from build123d import *

# Parameters (mm, degrees)
SKETCH1_W           = 51.8
SKETCH1_H           = 10.8
BOSS_EXTRUDE1_DEPTH = 12
BOSS_EXTRUDE2_DEPTH = 4
CUT_EXTRUDE1_DEPTH  = 36.675902231
FILLET1_R           = 1
SKETCH4_R           = 3.25
CUT_EXTRUDE2_DEPTH  = 36.675902231
SKETCH5_R           = 4
CUT_EXTRUDE3_DEPTH  = 1.05
M4_TAPPED_HOLE1_D   = 3.3
SKETCH8_R           = 1.25
CUT_EXTRUDE4_DEPTH  = 33.723233337
M4_TAPPED_HOLE2_D   = 3.3


with BuildPart() as part:
    # Sketch1 → Boss-Extrude1 (new body)
    with BuildSketch(Plane.XY):
        Rectangle(SKETCH1_W, SKETCH1_H)
    extrude(amount=BOSS_EXTRUDE1_DEPTH)

    # Sketch2 → Boss-Extrude2 (add)
    with BuildSketch(Plane.XY.offset(12)):
        with BuildLine():
            Line((-25.9, 14.9), (-25.9, 5.4))
            Line((-25.9, 5.4), (-12.9, 5.4))
            Line((-12.9, 5.4), (-12.9, 14.9))
            ThreePointArc((-12.9, 14.9), (-19.4, 21.4), (-25.9, 14.9))
        make_face()
    extrude(amount=-BOSS_EXTRUDE2_DEPTH)

    # Sketch3 → Cut-Extrude1 (cut, through all)
    with BuildSketch(Plane(origin=(0, 0, 0), x_dir=(-1, 0, 0), z_dir=(0, 0, -1))):
        with BuildLine():
            Line((-22.160417654, 0.869411765), (-25.9, 3.1))
            Line((-25.9, 3.1), (-25.9, -5.4))
            Line((-25.9, -5.4), (-18.6, -5.4))
            ThreePointArc((-18.6, -5.4), (-19.552207032, -1.795069427), (-22.160417654, 0.869411765))
        make_face()
    extrude(amount=-CUT_EXTRUDE1_DEPTH, mode=Mode.SUBTRACT)

    # Fillet1
    fillet1_edges = [part.edges().sort_by_distance(p)[0] for p in [
        (-25.9, 5.4, 4),
        (-12.9, 5.4, 10),
        (18.6, -5.4, 6),
        (25.9, 3.1, 6),
        (-25.9, -5.4, 6),
    ]]
    fillet(fillet1_edges, radius=FILLET1_R)

    # Sketch4 → Cut-Extrude2 (cut, through all)
    with BuildSketch(Plane(origin=(0, 0, 0), x_dir=(-1, 0, 0), z_dir=(0, 0, -1))):
        with Locations((20.65, 0.15)):
            Circle(SKETCH4_R)
    extrude(amount=-CUT_EXTRUDE2_DEPTH, mode=Mode.SUBTRACT)

    # Sketch5 → Cut-Extrude3 (cut)
    with BuildSketch(Plane(origin=(0, 0, 0), x_dir=(-1, 0, 0), z_dir=(0, 0, -1))):
        with Locations((20.65, 0.15)):
            Circle(SKETCH5_R)
    extrude(amount=-CUT_EXTRUDE3_DEPTH, mode=Mode.SUBTRACT)

    # M4 Tapped Hole1 (through all)
    with Locations(Plane(origin=(0, 5.4, 0), x_dir=(1, 0, 0), z_dir=(0, 1, 0))):
        with Locations((7.1, -6)):
            Hole(M4_TAPPED_HOLE1_D / 2)

    # Sketch8 → Cut-Extrude4 (cut, through all)
    with BuildSketch(Plane(origin=(0, 5.4, 0), x_dir=(1, 0, 0), z_dir=(0, 1, 0))):
        with Locations(Location((-11.9, -5.5, 0), (0, 0, 270))):
            Circle(SKETCH8_R)
    extrude(amount=-CUT_EXTRUDE4_DEPTH, mode=Mode.SUBTRACT)

    # M4 Tapped Hole2 (through all)
    with Locations(Plane.XY.offset(12)):
        with Locations((-18, 16.1)):
            Hole(M4_TAPPED_HOLE2_D / 2)


solid = part.part
Build history of the part. All positions in model axes, mm. A direction names the side the tool comes from. Coordinates: 2 decimals unless noted, no trailing zeros. Write each loop counter-clockwise with the first axis right and the second up, starting at its lowest first coordinate (ties: lowest second). Pieces come first, ordered by that corner, then holes.
(1) 3-axis set-ups, long thin cutter, end or side, ignore diameter. For faces 1 (the flat face through (-24, 2, 1.05)), 2 (the flat face through (0, 5.4, 6)), 3 (the flat face through (-12.9, 11, 10)): which of +Z, -Z, +X, -X, +Y, -Y reach the whole face in a straight line?
(2) Cut at A-A on x = 7.1. List the corners of the cut face in (y, z).
(3) Cut at B-B on y = -1.75. List the corners of the cut face in (x, z).
(4) Pin check, flat tips, straight feed: pin 1 Ø6 at (y, z) = (0, 6.5) entering from +X; pin 2 Ø6 at (x, z) = (3.5, 6.5) entering from +Y; pin 3 Ø7 at (x, y) = (-20.65, 0.15) entering from -Z. Stop position of each tip, or through.
(5) Mould opens along X. For faces 4 (the cylindrical face through (-13.12, 0.08, 5.23)), 5 (the flat face through (25.9, 5, 6)), 6 (the flat face through (0, 0, 0)), 7 (the cylindrical face through (-17.6, 14.5, 10)) say: pulls with the +X half, pulls with the -X half, needs draft (parallel to the pull), parting line crosses it, or undercut.
(6) Cut at D-D on y = 16.1. List the corners of the cut face in (x, z).
(7) Drill centre lines: line 1 (Z direction, x = 7.1, y = 0); line 2 (X direction, y = 4, z = 5); line 3 (Y direction, x = -20.65, z = 0.6). Where is each one in solid material? Low to high.
(8) Cut at C-C on z = 6. List the corners of the cut face in (x, y), and give its area (3 significant figures).
Working result:
1. face 1: -Z
1. face 2: -Z, +X, +Y
1. face 3: +Z, -Z, +X, +Y
2. outline: (-5.4, 0) - (5.4, 0) - (5.4, 4.35) - (-5.4, 4.35) - close; (-5.4, 7.65) - (5.4, 7.65) - (5.4, 12) - (-5.4, 12) - close
3. outline: (-25.9, 0) - (-24.17, 0) - (-24.17, 1.05) - (-23.29, 1.05) - (-23.29, 12) - (-25.9, 12) - close; (-18.01, 1.05) - (-17.13, 1.05) - (-17.13, 0) - (19.58, 0) - (19.58, 12) - (-18.01, 12) - close; hole circle Ø2.5 at (-11.9, 5.5); hole circle Ø3.3 at (7.1, 6)
4. pin 1: stops at x = 25.64
4. pin 2: stops at y = 5.4
4. pin 3: stops at z = 1.05
5. face 4: undercut
5. face 5: pulls with the +X half
5. face 6: needs draft
5. face 7: undercut
6. outline: (-25.79, 8) - (-19.65, 8) - (-19.65, 12) - (-25.79, 12) - close; (-16.35, 8) - (-13.01, 8) - (-13.01, 12) - (-16.35, 12) - close
7. line 1: z = 0 to 4.35, 7.65 to 12
7. line 2: x = -25.9 to -13.05, -10.75 to 5.79, 8.41 to 25.9
7. line 3: y = -5.4 to -3.85, 4.15 to 5.4
8. outline: (-25.9, -4.4) arc R1 ccw to (-24.9, -5.4) - (-13.05, -5.4) - (-13.05, 5.4) - (-24.9, 5.4) arc R1 ccw to (-25.9, 4.4) - close; (-10.75, -5.4) - (5.45, -5.4) - (5.45, 5.4) - (-10.75, 5.4) - close; (8.75, -5.4) - (17.66, -5.4) arc R1 ccw to (18.65, -4.52) arc R7.3 cw to (22.16, 0.87) - (25.41, 2.81) arc R1 ccw to (25.9, 3.67) - (25.9, 5.4) - (8.75, 5.4) - close; hole circle Ø6.5 at (-20.65, 0.15)
8. area: 422 mm2
